Autodesk Inventor part; units mm, degrees
ref_plane "YZ Plane" through (0, 0, 0) normal (1, 0, 0) x (0, 1, 0)
ref_plane "XZ Plane" through (0, 0, 0) normal (0, 1, 0) x (-1, 0, 0)
ref_plane "XY Plane" through (0, 0, 0) normal (0, 0, 1) x (1, 0, 0)
sketch "Sketch1" plane through (0, 0, 0) normal (0, 0, 1) x (1, 0, 0)
  line L0 (3, 0) -> (0, 0)
  line L1 (0, 0) -> (0, 9.7)
  line L2 (0, 9.7) -> (-6.163, 9.7)
  line L3 (-6.163, 9.7) -> (-6.163, 47.7)
  line L4 (-6.163, 47.7) -> (-3.163, 47.7)
  line L5 (-3.163, 47.7) -> (-3.163, 12.7)
  line L6 (-3.163, 12.7) -> (3, 12.7)
  line L7 (3, 12.7) -> (3, 3)
  line L8 (3, 3) -> (10.045, 3)
  line L9 (11.5096, 0) -> (9.0351, 0)
  line L10 (10.045, 3) -> (38, 3)
  line L11 (38, 3) -> (38, 0)
  line L12 (0, 0) -> (38, 0)
  point P0 (-3.0815, 9.7)
  dimension "d0" = 9.7
  dimension "d1" = 6.163
  dimension "d2" = 38
  dimension "d3" = 3
  dimension "d6" = 3
  dimension "d7" = 3
  dimension "d8" = 3
  dimension "d10" = 38
extrude "Extrusion1" add sketch "Sketch1" along normal blind 85
sketch "Sketch3" plane through (3, 3, 0) normal (1, 0, 0) x (0, 0, -1)
  point P0 (0, -3)
sketch "Sketch8" plane through (-3.163, 12.7, 0) normal (1, 0, 0) x (0, 0, -1)
  circle A0 centre (-76.25, 25.85) radius 2.1
  line L0 (-85, 0) -> (-85, 35)
  line L1 (0, 35) -> (-85, 35)
  point P0 (0, -12.7)
  dimension "d28" = 4.2
  dimension "d29" = 8.75
  dimension "d30" = 9.15
hole "Hole1" at (-3.163, 38.55, 76.25) direction (-1, 0, 0) diameter 4.2 end through all
sketch "Sketch9" plane through (-3.163, 12.7, 0) normal (1, 0, 0) x (0, 0, -1)
  circle A0 centre (-12.601, 25.85) radius 2.1
  line L0 (0, 35) -> (-85, 35)
  line L1 (0, 0) -> (0, 35)
  point P0 (0, -12.7)
  dimension "d38" = 4.2
  dimension "d39" = 9.15
  dimension "d40" = 12.601
hole "Hole2" at (-3.163, 38.55, 12.601) direction (-1, 0, 0) diameter 4.2 end through all
sketch "Sketch10" plane through (0, 0, 0) normal (0, -1, 0) x (1, 0, 0)
  line L0 (38, 0) -> (38, 85)
  line L1 (0, 0) -> (0, 85)
  line L2 (38, 25.2) -> (0, 25.2)
  line L3 (0, 25.2) -> (0, 49.2)
  line L4 (0, 49.2) -> (38, 49.2)
  line L5 (38, 49.2) -> (38, 25.2)
  line L6 (0, 0) -> (38, 0)
  line L7 (0, 85) -> (38, 85)
  point P0 (38, 49.2)
  point P1 (0, 25.2)
  dimension "d49" = 24
  dimension "d52" = 35.8
extrude "Extrusion7" cut sketch "Sketch10" against normal blind 3 contours L2 L1 L4 L0
sketch "Sketch12" plane through (3, 3, 85) normal (0, 1, 0) x (1, 0, 0)
  circle A0 centre (16.672, 16.473) radius 2.1
  line L0 (35, 0) -> (0, 0)
  line L1 (0, 35.8) -> (0, 0)
  point P0 (-3, 85)
  dimension "d63" = 4.2
  dimension "d64" = 16.473
  dimension "d65" = 16.672
hole "Hole4" at (19.672, 3, 68.527) direction (0, -1, 0) diameter 4.2 end through all
sketch "Sketch13" plane through (3, 3, 0) normal (0, 1, 0) x (1, 0, 0)
  circle A0 centre (16.672, -18.288) radius 2.1
  line L0 (0, 0) -> (0, -25.2)
  line L1 (35, 0) -> (0, 0)
  point P0 (-3, 0)
  dimension "d73" = 4.2
  dimension "d74" = 16.672
  dimension "d75" = 18.288
hole "Hole5" at (19.672, 3, 18.288) direction (0, -1, 0) diameter 4.2 end through all
sketch "Sketch14" plane through (3, 3, 0) normal (1, 0, 0) x (0, 0, -1)
  line L0 (-49.2, 0) -> (-85, 0)
  line L1 (0, 9.7) -> (-85, 9.7)
  line L2 (-49.2, 0) -> (-25.2, 0)
  line L3 (-25.2, 0) -> (-25.2, 9.7)
  line L4 (-25.2, 9.7) -> (-49.2, 9.7)
  line L5 (-49.2, 9.7) -> (-49.2, 0)
  point P0 (0, -3)
  point P1 (-49.2, 9.7)
  dimension "d83" = 24
extrude "Extrusion8" cut sketch "Sketch14" against normal blind 3.2
properties part number "RotaryActBracket"
CAD build for the part. Positions are in the model's coordinates, mm. A direction names the side the tool comes from. Round coordinates to 2 decimals unless told otherwise and drop trailing zeros. Order: outer loops, then holes, each group sorted by start corner. A loop starts at its lowest first (then second) coordinate and runs counter-clockwise, first axis right, second up.
Item 1: Pin check, flat tips, straight feed: pin 1 (1.5 mm diameter, centred on y = 10.5, z = 35, fed in from +X); pin 2 (1 mm diameter, centred on y = 32.5, z = 54.5, fed in from +X); pin 3 (1.5 mm diameter, centred on x = 21.5, z = 9.5, fed in from +Y). Stop position of each tip, or through.
Item 2: Mould opens along Z. For faces 4 (the face through (14.7, 2.6, 49.2)), 5 (the face through (2.7, 11.6, 85)), 6 (the face through (38, 2, 12)) say: pulls with the +Z half, pulls with the -Z half, needs draft (parallel to the pull), parting line crosses it, or undercut.
Item 3: Tool access for faces 1 (the face through (-1, 12.7, 42)), 2 (the face through (0, 5, 12)), 3 (the face through (-4.684, 39.828, 77.916)): list every direction of +Z, -Z, +X, -X, +Y, -Y with a clear straight run to the whole face (end or side of a thin tool).
Item 4: Saw through at B-B on y = 8.5. Write the cut outline in (x, z), then the cut area to 3 significant figures.
Item 5: Probe line 1 along Y through (x, z) = (-4, 76); line 2 along X through (y, z) = (43.5, 22); line 3 along Y through (x, z) = (35, 5). List the from-to ranges inside material, lowest first.
Item 6: Saw through at A-A on y = 38.55. Write the cut outline in (x, z), then the cut area to 3 significant figures.
Item 7: Saw through at D-D on z = 76.25. Write the cut outline in (x, y).
Reported:
1. pin 1: stops at x = -0.2
1. pin 2: stops at x = -3.16
1. pin 3: stops at y = 3
2. face 4: undercut
2. face 5: pulls with the +Z half
2. face 6: needs draft
3. face 1: +Z, -Z, +X, +Y
3. face 2: +Z, -Z, -X, -Y
3. face 3: +X, -X
4. outline: (0, 0) - (3, 0) - (3, 25.2) - (0, 25.2) - close; (0, 49.2) - (3, 49.2) - (3, 85) - (0, 85) - close
4. area: 183 mm2
5. line 1: y = 9.7 to 36.46, 40.64 to 47.7
5. line 2: x = -6.16 to -3.16
5. line 3: y = 0 to 3
6. outline: (-6.16, 0) - (-3.16, 0) - (-3.16, 10.5) - (-6.16, 10.5) - close; (-6.16, 14.7) - (-3.16, 14.7) - (-3.16, 74.15) - (-6.16, 74.15) - close; (-6.16, 78.35) - (-3.16, 78.35) - (-3.16, 85) - (-6.16, 85) - close
6. area: 230 mm2
7. outline: (-6.16, 9.7) - (0, 9.7) - (0, 0) - (38, 0) - (38, 3) - (3, 3) - (3, 12.7) - (-3.16, 12.7) - (-3.16, 36.45) - (-6.16, 36.45) - close; (-6.16, 40.65) - (-3.16, 40.65) - (-3.16, 47.7) - (-6.16, 47.7) - close
